For this review, use the dimensioned drawing (mm, ordinates from the lowest corner) and the shaded views. A direction names the side the tool comes from. Round coordinates to 2 decimals unless told otherwise and drop trailing zeros. Write each loop counter-clockwise with the first axis right and the second up, starting at its lowest first coordinate (ties: lowest second). Pieces come first, ordered by that corner, then holes. Notation, with made-up numbers: M -11,32.25 L 15,32.25 A17 cw 15,53.25 Z; hole C 61,46 d10. An arc over 180 degrees is marked long. Answer in a Markdown table with one row per item.
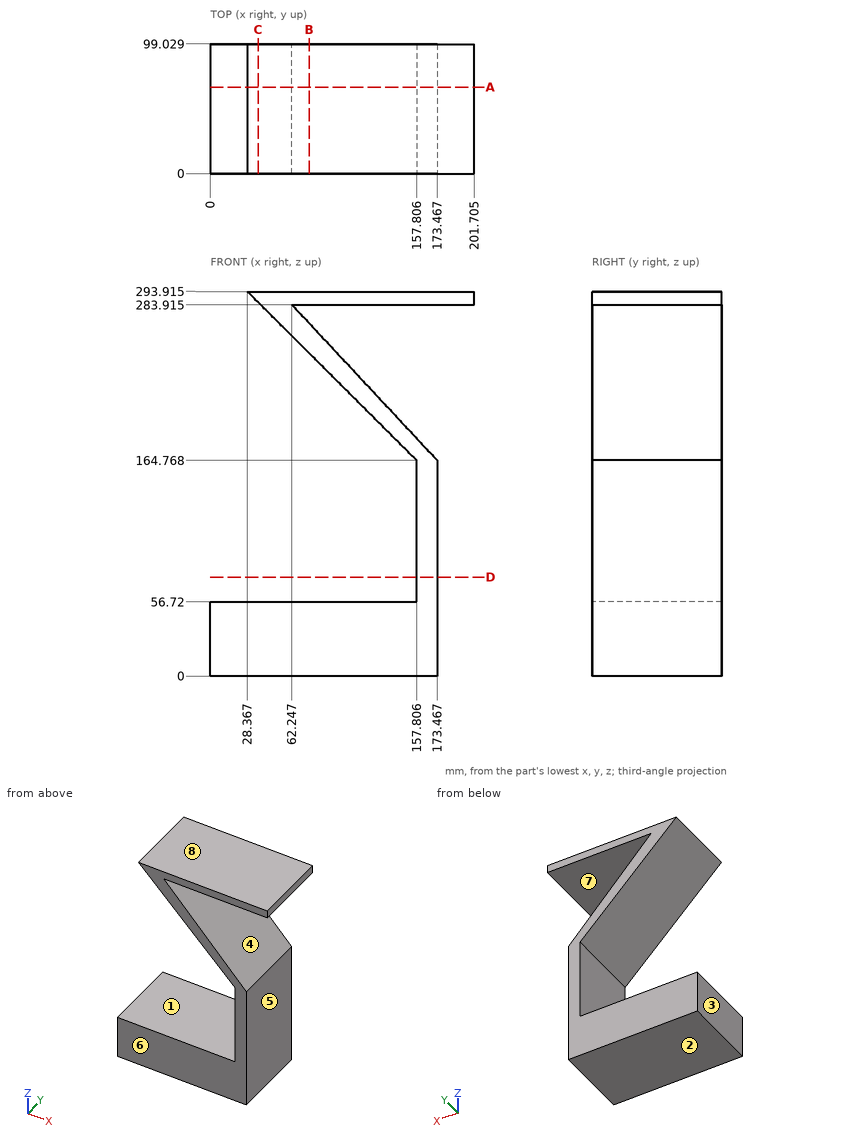
Q1. Mouldability with a two-part tool opening along Z and no side actions: class the marked faces 6, 7 and 8 as +Z half, -Z half, draft (parallel to the pull), parting line (faces both ways), or undercut.
Found:
| item | result |
|---|---|
| face 6 | draft |
| face 7 | undercut |
| face 8 | +Z half |
Q2. Take a section at A-A (y = 66). State the section outline as (x, z) points (1 decimal), then the cut area to 3 significant figures.
Found:
| item | result |
|---|---|
| outline | M 0,0 L 173.5,0 L 173.5,164.8 L 62.2,283.9 L 201.7,283.9 L 201.7,293.9 L 28.4,293.9 L 157.8,164.8 L 157.8,56.7 L 0,56.7 Z |
| area | 15,600 mm² |
Q3. Machinability: for the marked faces 1, 2, 3, 4 and 5, which of the approach directions +Z, -Z, +X, -X, +Y, -Y give a long, thin tool a straight path to every point of the face, cutting with its end or side? Answer none if there is none.
Found:
| item | result |
|---|---|
| face 1 | -X, +Y, -Y |
| face 2 | -Z, +X, -X, +Y, -Y |
| face 3 | +Z, -Z, -X, +Y, -Y |
| face 4 | +X, +Y, -Y |
| face 5 | -Z, +X, +Y, -Y |
Q4. Take a section at C-C (x = 36.5). State the section outline as (y, z) points (1 decimal).
Found:
| item | result |
|---|---|
| outline | M 0,0 L 99,0 L 99,56.7 L 0,56.7 Z; M 0,285.8 L 99,285.8 L 99,293.9 L 0,293.9 Z |
Q5. Take a section at D-D (z = 75.5). State the section outline as (x, y) points, then the cut area to 3 significant figures.
Found:
| item | result |
|---|---|
| outline | M 157.81,0 L 173.47,0 L 173.47,99.03 L 157.81,99.03 Z |
| area | 1,550 mm² |
Q6. Take a section at B-B (x = 75.5). State the section outline as (y, z) points (1 decimal), then the cut area to 3 significant figures.
Found:
| item | result |
|---|---|
| outline | M 0,0 L 99,0 L 99,56.7 L 0,56.7 Z; M 0,246.9 L 99,246.9 L 99,269.7 L 0,269.7 Z; M 0,283.9 L 99,283.9 L 99,293.9 L 0,293.9 Z |
| area | 8,870 mm² |
Q7. Insertion check: P1, Ø1, axis at y = 76, z = 37, coming from the +X side; P2, Ø12, axis at y = 19, z = 242, coming from the +X side (1 decimal); P3, Ø1.5, axis at y = 69, z = 228.5, coming from the -X side. Each pin has a flat end and moves straight along its axis. Give the tip position at first contact, or say it passes through.
Found:
| item | result |
|---|---|
| P1 | x = 173.47 |
| P2 | x = 107 |
| P3 | x = 93.18 |
Q8. For probe 1 along Z at (x, y) = (131, 79) (1 decimal); probe 2 along Z at (x, y) = (66, 49) (1 decimal); probe 3 along X at (y, z) = (12.5, 141), list the stretches that pass through material, from the lowest coordinate up.
Found:
| item | result |
|---|---|
| probe 1 | 0 to 56.7, 191.5 to 210.3, 283.9 to 293.9 |
| probe 2 | 0 to 56.7, 256.4 to 279.9, 283.9 to 293.9 |
| probe 3 | 157.81 to 173.47 |
